Geometry check sheet. Reference: the model listing, model coordinates, mm. A direction names the side the tool comes from. Give positions to 0.01 mm unless a question says otherwise; leave off trailing zeros. Write each loop counter-clockwise with the first axis right and the second up, starting at its lowest first coordinate (ties: lowest second). Pieces come first, ordered by that corner, then holes. Notation, with made-up numbers: M -35,3.5 L 10,3.5 A22 cw 10,11.5 Z; hole C 51.5,17 d8. An arc over 180 degrees is marked long. One line per item, written item: value. Start each with the question number.
1. Cross-section at D-D on x = 24. Record the cut outline in (y, z), then the cut area to 3 significant figures.
2. Release check for a two-part mould opening along Z. For faces 1 (the face through (13.2, 39.144, 12.3)), 2 (the face through (24.74, 35.87, 3.6)), 3 (the face through (8.3, 28.17, 0.22)) record: pulls with the +Z half, pulls with the -Z half, needs draft (parallel to the pull), parting line crosses it, or undercut.
3. Gauge pin test, flat ends, axial feed: pin 1 (1 mm diameter, centred on x = 6, y = 20.5, fed in from -Z); pin 2 (3 mm diameter, centred on y = 33, z = -8, fed in from +X); pin 3 (3 mm diameter, centred on y = 30, z = -4.5, fed in from -X). Record the tip position at first contact, or that the pin passes through.
4. Scan lines: line 1 (Y direction, x = 25.5, z = -1.75); line 2 (Z direction, x = 13.5, y = 20.5); line 3 (X direction, y = 37.5, z = 1.5). Record each from-to range of solid material in increasing order.
5. Cross-section at B-B on x = 10.5. Record the cut outline in (y, z).
6. Cross-section at C-C on y = 36.5. Record the cut outline in (x, z), then the cut area to 3 significant figures.
7. Tool access check on faces 4 (the face through (-1.69, 29.87, 0.66)), 5 (the face through (13.2, 27.122, 12.3)). Record the directions out of +Z, -Z, +X, -X, +Y, -Y that give a thin tool (end or side, any length) a straight path to the whole face; none if there is none.
8. Cross-section at A-A on z = 0. Record the cut outline in (x, y).
Autodesk Fusion 360 part; units mm, degrees
sketch "Sketch1" plane through (0, 0, 0) normal (0, 0, 1) x (1, 0, 0)
  line L0 (18.2937, 44.1436) -> (28.2937, 44.1436)
  line L1 (28.2937, 44.1436) -> (28.2937, 39.1436)
  line L2 (28.2937, 39.1436) -> (25.2937, 39.1436)
  line L3 (25.2937, 39.1436) -> (25.2937, 32.6901)
  line L4 (25.2937, 32.6901) -> (28.2937, 32.6901)
  line L5 (28.2937, 32.6901) -> (28.2937, 27.1224)
  line L6 (28.2937, 27.1224) -> (25.2937, 27.1224)
  line L7 (25.2937, 27.1224) -> (25.2937, 22.9865)
  line L8 (25.2937, 22.9865) -> (28.2937, 22.9865)
  line L9 (28.2937, 22.9865) -> (28.2937, 12.6465)
  line L10 (18.2937, 44.1436) -> (18.2937, 12.6465)
  line L11 (28.2937, 12.6465) -> (18.2937, 12.6465)
  line L12 (13.2937, 44.1436) -> (13.2937, 53)
  dimension "d1" = 10
  dimension "d2" = 5
  dimension "d3" = 3
  dimension "d4" = 5
revolve "Revolve2" add sketch "Sketch1" angle 360 about axis through (13.2937, 53, 0) along (0, -1, 0)
Report:
1. outline: M 12.65,-10.51 L 22.99,-10.51 L 22.99,-5.42 L 27.12,-5.42 L 27.12,-10.51 L 32.69,-10.51 L 32.69,-5.42 L 39.14,-5.42 L 39.14,-10.51 L 44.14,-10.51 L 44.14,10.51 L 39.14,10.51 L 39.14,5.42 L 32.69,5.42 L 32.69,10.51 L 27.12,10.51 L 27.12,5.42 L 22.99,5.42 L 22.99,10.51 L 12.65,10.51 Z
1. area: 554 mm^2
2. face 1: needs draft
2. face 2: parting line crosses it
2. face 3: undercut
3. pin 1: stops at z = -13.37
3. pin 2: stops at x = 26.8
3. pin 3: stops at x = -1.4
4. line 1: y = 12.65 to 22.99, 27.12 to 32.69, 39.14 to 44.14
4. line 2: z = -15 to -5, 5 to 15
4. line 3: x = 1.39 to 8.52, 18.06 to 25.2
5. outline: M 12.65,-14.74 L 22.99,-14.74 L 22.99,-11.67 L 27.12,-11.67 L 27.12,-14.74 L 32.69,-14.74 L 32.69,-11.67 L 39.14,-11.67 L 39.14,-14.74 L 44.14,-14.74 L 44.14,-4.15 L 12.65,-4.15 Z; M 12.65,4.15 L 44.14,4.15 L 44.14,14.74 L 39.14,14.74 L 39.14,11.67 L 32.69,11.67 L 32.69,14.74 L 27.12,14.74 L 27.12,11.67 L 22.99,11.67 L 22.99,14.74 L 12.65,14.74 Z
6. outline: C 13.29,0 d24; hole C 13.29,0 d10
6. area: 374 mm^2
7. face 4: +Y, -Y
7. face 5: none
8. outline: M -1.71,12.65 L 8.29,12.65 L 8.29,44.14 L -1.71,44.14 L -1.71,39.14 L 1.29,39.14 L 1.29,32.69 L -1.71,32.69 L -1.71,27.12 L 1.29,27.12 L 1.29,22.99 L -1.71,22.99 Z; M 18.29,12.65 L 28.29,12.65 L 28.29,22.99 L 25.29,22.99 L 25.29,27.12 L 28.29,27.12 L 28.29,32.69 L 25.29,32.69 L 25.29,39.14 L 28.29,39.14 L 28.29,44.14 L 18.29,44.14 Z
